```python
from build123d import *

# Parameters (mm, degrees)
SZKIC5_R                   = 3.2
WYTNIJ_WYCI_GNI_CIE1_DEPTH = 19


with BuildPart() as part:
    # Szkic1 → Obrót1 (revolve)
    with BuildSketch(Plane.XY, mode=Mode.PRIVATE) as obr_t1_sk:
        with BuildLine():
            Line((0, -16.5), (1, -17.5))
            Line((1, -17.5), (4.4, -17.5))
            Line((4.4, -17.5), (5.4, -16.5))
            Line((5.4, -16.5), (9.78348732, -16.5))
            ThreePointArc((9.78348732, -16.5), (10.913937759, -16.070336685), (11.473614893, -14.998287122))
            ThreePointArc((11.473614893, -14.998287122), (11.326095192, -13.919522313), (10.672757631, -13.048519668))
            Line((10.672757631, -13.048519668), (6.370526458, -9.966460766))
            ThreePointArc((6.370526458, -9.966460766), (5.5, -8.24315268), (6.348844005, -6.509061873))
            Line((6.348844005, -6.509061873), (10.670037967, -3.453646536))
            ThreePointArc((10.670037967, -3.453646536), (11.32543403, -2.582085517), (11.473614893, -1.501712878))
            ThreePointArc((11.473614893, -1.501712878), (10.913937759, -0.429663315), (9.78348732, 0))
            Line((9.78348732, 0), (5.4, 0))
            Line((5.4, 0), (4.4, 1))
            Line((4.4, 1), (1, 1))
            Line((1, 1), (0, 0))
            Line((0, 0), (-3.2, 0))
            Line((-3.2, 0), (-3.2, -16.5))
            Line((-3.2, -16.5), (0, -16.5))
        make_face()
    revolve(obr_t1_sk.sketch.rotate(Axis((-3.2, 0, 0), (0, -1, 0)), 180), axis=Axis((-3.2, 0, 0), (0, -1, 0)))

    # Szkic5 → Wytnij-wyciągnięcie1 (cut)
    with BuildSketch(Plane(origin=(0, 0, 0), x_dir=(1, 0, 0), z_dir=(0, 1, 0))):
        with Locations(Location((-3.2, 0, 0), (0, 0, 180))):
            Circle(SZKIC5_R)
    extrude(amount=-WYTNIJ_WYCI_GNI_CIE1_DEPTH, mode=Mode.SUBTRACT)


solid = part.part
```
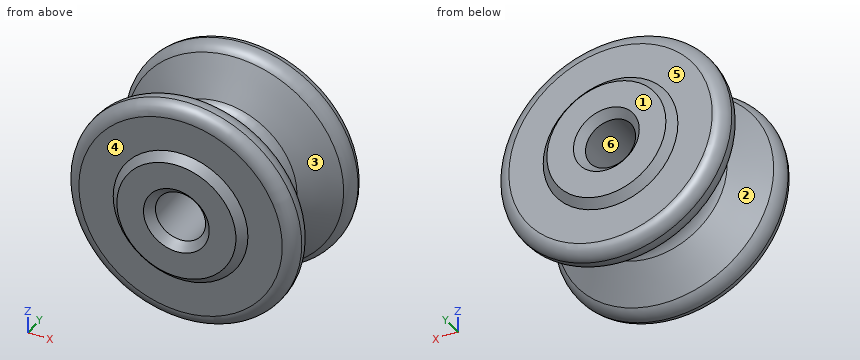
Work out the finished part from the listing and answer in its coordinate system (mm). Face numbers are marked on the shaded views. A direction names the side the tool comes from. Coordinates: 2 decimals unless noted, no trailing zeros. Write each loop counter-clockwise with the first axis right and the second up, starting at its lowest first coordinate (ties: lowest second). Pieces come first, ordered by that corner, then holes.
Q1. Find the intervals of material crossed by line 1 (Z direction, x = -3.2, y = -6.5); line 2 (X direction, y = -15, z = -1.25); line 3 (Y direction, x = -12.5, z = 1.25), in increasing order.
Q2. Which of the six approach directions +Z, -Z, +X, -X, +Y, -Y give full straight-line access (tool end or side, diameter ignored) to the marked faces 5 and 6?
Q3. Determine the mould class of the marked faces 1, 2, 3 and 4 for opening direction Y: released by +Y, released by -Y, zero draft, split by the parting line, or undercut.
Q4. Each of these flat-tipped pins is pushed along its axis until it touches: pin 1 Ø5 at (x, z) = (-12.5, -4.5) entering from -Y; pin 2 Ø1 at (y, z) = (-7, -3) entering from -X; pin 3 Ø4 at (x, y) = (7, -2.5) entering from -Z. Where does it stop, or does it pass through?
Q5. A cutting plane is placed at C-C, the plane y = -2.25. Give the vertices of the cut face in (x, z).
Findings below:
1. line 1: z = -9.56 to -3.2, 3.2 to 9.56
1. line 2: x = -17.82 to -6.15, -0.25 to 11.42
1. line 3: y = -16.5 to -9.81, -6.65 to 0
2. face 5: +Y
2. face 6: +Y, -Y
3. face 1: released by +Y
3. face 2: undercut
3. face 3: undercut
3. face 4: released by -Y
4. pin 1: stops at y = -17.27
4. pin 2: stops at x = -12.3
4. pin 3: stops at z = -12.13
5. outline: circle Ø29.26 at (-3.2, 0); hole circle Ø6.4 at (-3.2, 0)
